The listing builds one solid part. Answer for the finished solid, in the listing's coordinates (mm). A direction names the side the tool comes from. Coordinates: 2 decimals unless noted, no trailing zeros. Write each loop counter-clockwise with the first axis right and the second up, starting at its lowest first coordinate (ties: lowest second). Pieces come first, ordered by that corner, then holes. Notation, with made-up numbers: M 14.5,-16.5 L 26.5,-16.5 A9 cw 26.5,-7.5 Z; hole C 57,10.25 d5. An arc over 180 degrees is marked long. Answer as CSV lines item,"result".
```python
from build123d import *

# Parameters (mm, degrees)
ESBO_O1_W                = 67
ESBO_O1_H                = 62
RESSALTO_EXTRUS_O1_DEPTH = 15
ESBO_O2_R                = 2.5
ESBO_O2_R_2              = 2
CORTE_EXTRUS_O1_DEPTH    = 93.509458976
ESBO_O3_W                = 62
ESBO_O3_H                = 15
RESSALTO_EXTRUS_O2_DEPTH = 30
ESBO_O4_R                = 2.5
CORTE_EXTRUS_O2_DEPTH    = 93.509458976
ESBO_O5_R                = 4
CORTE_EXTRUS_O3_DEPTH    = 5


with BuildPart() as part:
    # Esboço1 → Ressalto-extrusão1 (new body)
    with BuildSketch(Plane(origin=(0, 0, 0), x_dir=(1, 0, 0), z_dir=(0, 1, 0))):
        with Locations((33.5, -31)):
            Rectangle(ESBO_O1_W, ESBO_O1_H)
    extrude(amount=RESSALTO_EXTRUS_O1_DEPTH)

    # Esboço2 → Corte-extrusão1 (cut, through all)
    with BuildSketch(Plane(origin=(0, 15, 0), x_dir=(1, 0, 0), z_dir=(0, 1, 0))):
        with Locations(Location((60, -13.3, 0), (0, 0, 270))):
            Circle(ESBO_O2_R)
        with Locations(Location((60, -48.7, 0), (0, 0, 270))):
            Circle(ESBO_O2_R)
        with Locations(Location((29, -46.5, 0), (0, 0, 270))):
            Circle(ESBO_O2_R_2)
        with Locations(Location((28.970556633, -31, 0), (0, 0, 270))):
            Circle(ESBO_O2_R_2)
        with Locations(Location((29, -15.5, 0), (0, 0, 270))):
            Circle(ESBO_O2_R_2)
    extrude(amount=-CORTE_EXTRUS_O1_DEPTH, mode=Mode.SUBTRACT)

    # Esboço3 → Ressalto-extrusão2 (add)
    with BuildSketch(Plane.ZY):
        with Locations((31, 7.5)):
            Rectangle(ESBO_O3_W, ESBO_O3_H)
    extrude(amount=RESSALTO_EXTRUS_O2_DEPTH)

    # Esboço4 → Corte-extrusão2 (cut, through all)
    with BuildSketch(Plane(origin=(0, 15, 0), x_dir=(1, 0, 0), z_dir=(0, 1, 0))):
        with Locations(Location((-15, -31, 0), (0, 0, 270))):
            Circle(ESBO_O4_R)
        with Locations(Location((-15, -6.93, 0), (0, 0, 270))):
            Circle(ESBO_O4_R)
        with Locations(Location((-15, -55.07, 0), (0, 0, 270))):
            Circle(ESBO_O4_R)
    extrude(amount=-CORTE_EXTRUS_O2_DEPTH, mode=Mode.SUBTRACT)

    # Esboço5 → Corte-extrusão3 (cut)
    with BuildSketch(Plane(origin=(0, 15, 0), x_dir=(1, 0, 0), z_dir=(0, 1, 0))):
        with Locations(Location((-15, -6.93, 0), (0, 0, 270))):
            Circle(ESBO_O5_R)
        with Locations(Location((-15, -31, 0), (0, 0, 270))):
            Circle(ESBO_O5_R)
        with Locations(Location((-15, -55.07, 0), (0, 0, 270))):
            Circle(ESBO_O5_R)
    extrude(amount=-CORTE_EXTRUS_O3_DEPTH, mode=Mode.SUBTRACT)


solid = part.part
```
Q1. The mould has two halves that part along Z. Classify faces 1 (the flat face through (19, 15, 31)), 2 (the flat face through (19, 7, 0)), 3 (the cylindrical face through (-14.824, 12.535, 51.074)): pulls with the +Z half, pulls with the -Z half, needs draft (parallel to the pull), parting line crosses it, or undercut.
Output:
face 1,"needs draft"
face 2,"pulls with the -Z half"
face 3,"undercut"
Q2. For faces 4 (the flat face through (-17, 10, 53)), 5 (the cylindrical face through (27.048, 7.605, 46.066)), determine the directions among +Z, -Z, +X, -X, +Y, -Y from which every point of the face is accessible in a straight line to the end or side of a thin tool.
Output:
face 4,"+Y"
face 5,"+Y, -Y"
Q3. Find section A-A (z = 55.07). Give the vertices of the cut face in (x, y).
Output:
outline,"M -30,0 L -17.5,0 L -17.5,10 L -19,10 L -19,15 L -30,15 Z; M -12.5,0 L 67,0 L 67,15 L -11,15 L -11,10 L -12.5,10 Z"
Q4. A flat-ended cylindrical pin translates along its axis: pin 1 Ø6 at (x, z) = (-15, 31) entering from +Y. Find the tip coordinate at first contact, or state that the pin passes through.
Output:
pin 1,"y = 10"
Q5. Find section B-B (x = 60). Give the vertices of the cut face in (y, z), and give its area (3 significant figures).
Output:
outline,"M 0,0 L 15,0 L 15,10.8 L 0,10.8 Z; M 0,15.8 L 15,15.8 L 15,46.2 L 0,46.2 Z; M 0,51.2 L 15,51.2 L 15,62 L 0,62 Z"
area,"780 mm2"
Q6. Straight lines are drawn through the part: line 1 (X direction, y = 13.75, z = 6.93); line 2 (X direction, y = 5.5, z = 55.07); line 3 (X direction, y = 4.25, z = 31). For each, find the intervals that lie inside material, in ascending order.
Output:
line 1,"-30 to -19, -11 to 67"
line 2,"-30 to -17.5, -12.5 to 67"
line 3,"-30 to -17.5, -12.5 to 26.97, 30.97 to 67"
Q7. Find section C-C (y = 1). Count the separate pieces of the cut face and the enclosed holes in it, and give its area (3 significant figures).
Output:
separate pieces,"1"
enclosed holes,"8"
area,"5,880 mm2"
